from build123d import *

# Parameters (mm, degrees)
F0_R   = 4
F0_R_2 = 3.75
F3_R   = 3.9


with BuildPart() as f2:
    # F2: sweep along a path in F1
    with BuildLine(Plane.XY) as f2_path:
        Line((0, 0), (0, 40))
    # F0 (on Front) → F2 (sweep)
    with BuildSketch(Plane.XZ):
        Circle(F0_R)
        Circle(F0_R_2, mode=Mode.SUBTRACT)
    sweep(path=f2_path.line)

    # F5: sweep along a path in F4
    with BuildLine(Plane.YZ) as f5_path:
        Line((21.1965255439, 0), (21.1965255439, 30))
    # F3 (on Top) → F5 (sweep, cut)
    with BuildSketch(Plane.XY):
        with Locations((0, 19.8551610578)):
            Circle(F3_R)
    sweep(path=f5_path.line, mode=Mode.SUBTRACT)


solid = f2.part
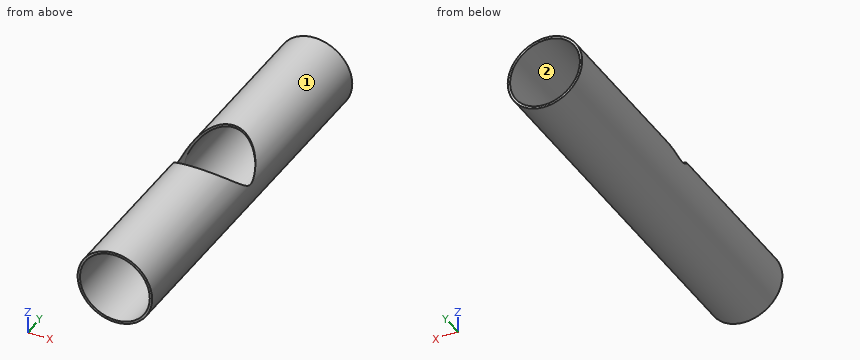
Verification items for the finished model (mm, model axes). Face numbers are marked on the shaded views. Coordinates: 2 decimals unless noted, no trailing zeros. Order: outer loops, then holes, each group sorted by start corner. A loop starts at its lowest first (then second) coordinate and runs counter-clockwise, first axis right, second up. Notation, with made-up numbers: M 5.5,-18 L 14.5,-18 A31 ccw 14.5,12 Z; hole C -27,12.5 d8. An arc over 180 degrees is marked long. One line per item, written item: value. Start each with the question number.
Item 1: Sectioned sample at C-C (z = 1.5). Enter the section's corners in (x, y), then the cut area to 3 significant figures.
Item 2: Sectioned sample at D-D (y = 5). Enter the section's corners in (x, z), then the cut area to 3 significant figures.
Item 3: Sectioned sample at A-A (x = 0). Enter the section's corners in (y, z), then the cut area to 4 significant figures.
Item 4: Scan lines: probe 1 along X at (y, z) = (27.5, 0); probe 2 along Z at (x, y) = (0, 23). Record each from-to range of solid material in increasing order.
Item 5: Gauge pin test, flat end, axial feed: pin 1 (1.5 mm diameter, centred on y = 33, z = 3, fed in from +X). Record the tip position at first contact, or that the pin passes through.
Item 6: Mould release check, pull along X, two halves, no side actions. Record for the marked faces 1 and 2: released by +X, released by -X, zero draft, split by the parting line, or undercut.
Item 7: Sectioned sample at B-B (z = -2). Enter the section's corners in (x, y).
Conclusion:
1. outline: M -3.71,0 L -3.44,0 L -3.44,18.01 A3.9 cw -3.71,18.65 Z; M -3.71,21.06 A3.9 cw -3.44,21.7 L -3.44,40 L -3.71,40 Z; M 3.44,0 L 3.71,0 L 3.71,18.65 A3.9 cw 3.44,18.01 Z; M 3.44,21.7 A3.9 cw 3.71,21.06 L 3.71,40 L 3.44,40 Z
1. area: 20.0 mm^2
2. outline: C 0,0 d8; hole C 0,0 d7.5
2. area: 6.09 mm^2
3. outline: M 0,-4 L 40,-4 L 40,-3.75 L 0,-3.75 Z; M 0,3.75 L 15.96,3.75 L 15.96,4 L 0,4 Z; M 23.76,3.75 L 40,3.75 L 40,4 L 23.76,4 Z
3. area: 18.05 mm^2
4. probe 1: x = -4 to -3.75, 3.75 to 4
4. probe 2: z = -4 to -3.75
5. pin 1: stops at x = 3.31
6. face 1: split by the parting line
6. face 2: undercut
7. outline: M -3.46,0 L -3.17,0 L -3.17,40 L -3.46,40 Z; M 3.17,0 L 3.46,0 L 3.46,40 L 3.17,40 Z
